```python
from build123d import *

# Parameters (mm, degrees)
SZKIC1_R                    = 6.5
SZKIC1_R_2                  = 3
DODANIE_WYCI_GNI_CIE1_DEPTH = 10


with BuildPart() as part:
    # Szkic1 → Dodanie-wyciągnięcie1 (new body)
    with BuildSketch(Plane.XY):
        with BuildLine():
            ThreePointArc((1.536461967, 29.061275164), (0.036461967, 27.561275164), (-1.463538033, 29.061275164))
            Line((-1.463538033, 29.061275164), (-1.463538033, 30.464865935))
            ThreePointArc((-1.463538033, 30.464865935), (-21.042957135, -22.07813296), (30.5, 0))
            ThreePointArc((30.5, 0), (22.103303938, 21.016516243), (1.536461967, 30.461275164))
            Line((1.536461967, 30.461275164), (1.536461967, 29.061275164))
        make_face()
        with Locations((-7.592965435, -15.766955188)):
            Circle(SZKIC1_R, mode=Mode.SUBTRACT)
        with Locations((-17.061238463, -3.894116344)):
            Circle(SZKIC1_R, mode=Mode.SUBTRACT)
        with Locations((7.592965435, -15.766955188)):
            Circle(SZKIC1_R, mode=Mode.SUBTRACT)
        with Locations((17.061238463, -3.894116344)):
            Circle(SZKIC1_R, mode=Mode.SUBTRACT)
        with Locations((-13.682050943, 10.911071533)):
            Circle(SZKIC1_R, mode=Mode.SUBTRACT)
        Circle(SZKIC1_R_2, mode=Mode.SUBTRACT)
        with Locations((13.682050943, 10.911071533)):
            Circle(SZKIC1_R, mode=Mode.SUBTRACT)
        with Locations((0, 17.5)):
            Circle(SZKIC1_R, mode=Mode.SUBTRACT)
    extrude(amount=DODANIE_WYCI_GNI_CIE1_DEPTH)


solid = part.part
```
Input: part model. Units: mm. Frame: model coordinates. A direction names the side the tool comes from. Coordinates: 2 decimals unless noted, no trailing zeros. Loops run counter-clockwise (first coordinate to the right, second up) from the corner with the lowest first, then second, coordinate; pieces in that order, holes last. Notation, with made-up numbers: M 75,56.25 L 113,56.25 A4 cw 113,60.25 Z; hole C 50,-13.75 d4. An arc over 180 degrees is marked long. Use a Markdown table: item, result. Add a question column.
1) Set-up query: faces 4 (the cylindrical face through (-20.176, 11.197, 4.93)), 5 (the flat face through (1.536, 30, 5)). Return all of +Z, -Z, +X, -X, +Y, -Y with unobstructed straight access to the full face (end or side cutting, diameter ignored); none if empty.
2) Section D-D, the plane z = 3. Give the number of separate pieces and of enclosed holes in the cut face, plus the area to 3 significant figures.
3) Section C-C, the plane x = 8. Return the cut outline in (y, z), plus the area to 3 significant figures.
4) Pin query (flat end, axial travel): P1, Ø1.5, axis at y = -17, z = 6.5, coming from the +X side; P2, Ø6, axis at x = 13, z = 3.5, coming from the -Y side; P3, Ø5, axis at x = -2, z = 2, coming from the +Y side; P4, Ø1.5, axis at x = -18, z = 4.5, coming from the -Y side. Return the tip coordinate at first contact, or that it passes through.
5) Section A-A, the plane y = -21. Return the cut outline in (x, z).
6) Line query: L1, parallel to Y at x = 0, z = 6; L2, parallel to Y at x = 14.5, z = 6; L3, parallel to X at y = 11.5, z = 4.5. Output: solid intervals per line, ascending. Write a range as from..to.
7) Draft query along Y for faces 1 (the flat face through (6, 0, 0)), 2 (the cylindrical face through (-22.22, -7.85, 4.93)), 3 (the cylindrical face through (0.07, 27.56, 4.93)). Return one class per face: +Y half, -Y half, draft (parallel to the pull), parting line (faces both ways), or undercut.
8) Section B-B, the plane y = 16. Return the cut outline in (x, z), plus the area to 3 significant figures.
Answer below:
| question | item | result |
|---|---|---|
| 1 | face 4 | +Z, -Z |
| 1 | face 5 | +Z, -Z, +Y |
| 2 | separate pieces | 1 |
| 2 | enclosed holes | 8 |
| 2 | area | 1,960 mm2 |
| 3 | outline | M -29.43,0 L -22.25,0 L -22.25,10 L -29.43,10 Z; M -9.28,0 L 7.75,0 L 7.75,10 L -9.28,10 Z; M 14.07,0 L 29.43,0 L 29.43,10 L 14.07,10 Z |
| 3 | area | 396 mm2 |
| 4 | P1 | x = 25.81 |
| 4 | P2 | y = -28.81 |
| 4 | P3 | y = 30.46 |
| 4 | P4 | y = -25.15 |
| 5 | outline | M -22.12,0 L -11.45,0 L -11.45,10 L -22.12,10 Z; M -3.74,0 L 3.74,0 L 3.74,10 L -3.74,10 Z; M 11.45,0 L 22.12,0 L 22.12,10 L 11.45,10 Z |
| 6 | L1 | -30.5..-3, 3..11, 24..27.56 |
| 6 | L2 | -26.83..-9.87, 2.08..4.46, 17.36..26.83 |
| 6 | L3 | -28.25..-20.16, -7.21..-2.5, 2.5..7.21, 20.16..28.25 |
| 7 | face 1 | draft |
| 7 | face 2 | undercut |
| 7 | face 3 | +Y half |
| 8 | outline | M -25.97,0 L -17.73,0 L -17.73,10 L -25.97,10 Z; M -9.64,0 L -6.32,0 L -6.32,10 L -9.64,10 Z; M 6.32,0 L 9.64,0 L 9.64,10 L 6.32,10 Z; M 17.73,0 L 25.97,0 L 25.97,10 L 17.73,10 Z |
| 8 | area | 231 mm2 |
